Read the model definition and answer for the solid it produces. Units are mm, in the model's axes. Face numbers are marked on the shaded views. A direction names the side the tool comes from. Coordinates: 2 decimals unless noted, no trailing zeros. Loops run counter-clockwise (first coordinate to the right, second up) from the corner with the lowest first, then second, coordinate; pieces in that order, holes last. Notation, with made-up numbers: (15, -1) - (34, -1) arc R19 cw to (34, 6) - close; hole circle Ø6 at (22, 87.25). An arc over 180 degrees is marked (long way). Use one line per item in the form item = value.
Autodesk Inventor part; units mm, degrees
ref_plane "YZ Plane" through (0, 0, 0) normal (1, 0, 0) x (0, 1, 0)
ref_plane "XZ Plane" through (0, 0, 0) normal (0, 1, 0) x (-1, 0, 0)
ref_plane "XY Plane" through (0, 0, 0) normal (0, 0, 1) x (1, 0, 0)
sketch "Sketch1" plane through (0, 0, 0) normal (0, 0, 1) x (1, 0, 0)
  circle A0 centre (0, 0) radius 11.1125
  dimension "d0" = 22.225
extrude "Extrusion1" add sketch "Sketch1" along normal blind 255.27
sketch "Sketch2" plane through (0, 0, 255.27) normal (0, 0, 1) x (1, 0, 0)
  line L0 (16.6687, 28.8711) -> (33.3375, 0)
  line L1 (33.3375, 0) -> (16.6687, -28.8711)
  line L2 (16.6687, -28.8711) -> (-16.6688, -28.8711)
  line L3 (-16.6688, -28.8711) -> (-33.3375, 0)
  line L4 (-33.3375, 0) -> (-16.6688, 28.8711)
  line L5 (-16.6688, 28.8711) -> (16.6687, 28.8711)
  circle A0 centre (0, 0) radius 11.1125 construction
  dimension "d3" = 33.3375
  dimension "d6" = 22.225
extrude "Extrusion2" add sketch "Sketch2" along normal blind 19.05
sketch "Sketch3" plane through (0, 0, 0) normal (0, 1, 0) x (-1, 0, 0)
  line L0 (33.3375, 274.32) -> (16.6687, 274.32)
  line L1 (29.5275, 274.32) -> (33.3375, 271.78)
  line L2 (33.3375, 271.78) -> (33.3375, 274.32)
  line L3 (33.3375, 274.32) -> (29.5275, 274.32)
  line L4 (0, -55.626) -> (0, 333.756)
  point P0 (0, 0)
  dimension "d7" = 2.54
  dimension "d8" = 3.81
revolve "Revolution1" cut sketch "Sketch3" angle 360 about axis through (0, 0, -10) along (0, 0, 1)
sketch "Sketch4" plane through (0, 0, 255.27) normal (0, 0, -1) x (-1, 0, 0)
  circle A0 centre (0, 0) radius 22.225
  dimension "d10" = 44.45
extrude "Extrusion3" add sketch "Sketch4" along normal blind 1.27
chamfer "Chamfer1" distance 3.175 angle 45 1 edges at (-11.1125, 0, 0)
thread "Thread1"
equation "\"d3\" = 1.5 * d6"
properties part number "HexBoltAJB" material "Iron, Malleable"
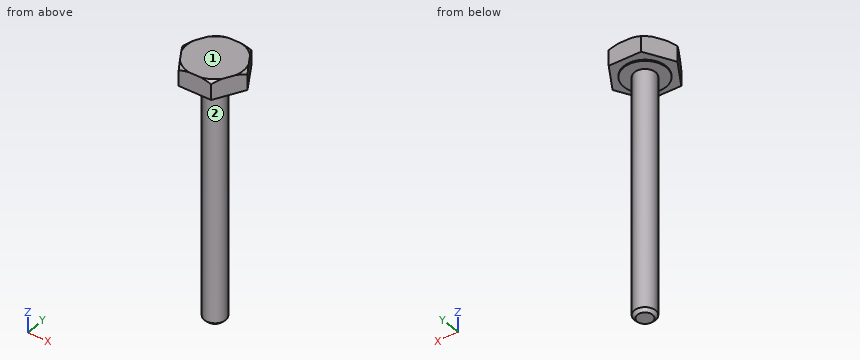
Item 1: Each of these flat-tipped pins is pushed along its axis until it touches: P1, Ø6, axis at x = 9.5, z = 80, coming from the +Y side; P2, Ø12, axis at y = 14, z = 65, coming from the +X side; P3, Ø5, axis at x = -3, z = 181.5, coming from the +Y side. Where does it stop, or does it pass through?
Results below:
P1 = 9.01
P2 = 7.71
P3 = 11.1
Item 2: The part is cut by section A-A on x = 0. Give the vertices of the cut face in (y, z) (1 decimal).
Results below:
outline = (-28.9, 255.3) - (-22.2, 255.3) - (-22.2, 254) - (-11.1, 254) - (-11.1, 3.2) - (-7.9, 0) - (7.9, 0) - (11.1, 3.2) - (11.1, 254) - (22.2, 254) - (22.2, 255.3) - (28.9, 255.3) - (28.9, 274.3) - (-28.9, 274.3) - close
Item 3: Find the intervals of material crossed by L1, parallel to Z at x = -0.5, y = -14; L2, parallel to Z at x = -25, y = 0.5; L3, parallel to X at y = -6.5, z = 112, in increasing order.
Results below:
L1 = 254 to 274.32
L2 = 255.27 to 274.32
L3 = -9.01 to 9.01
Item 4: The part is cut by section B-B on z = 52. Give the vertices of the cut face in (x, y) (1 decimal), plus the area to 3 significant figures.
Results below:
outline = circle Ø22.2 at (0, 0)
area = 388 mm²
Item 5: Which of the six approach directions +Z, -Z, +X, -X, +Y, -Y give full straight-line access (tool end or side, diameter ignored) to the marked faces 1 and 2?
Results below:
face_1 = +Z, +X, -X, +Y, -Y
face_2 = -Z
